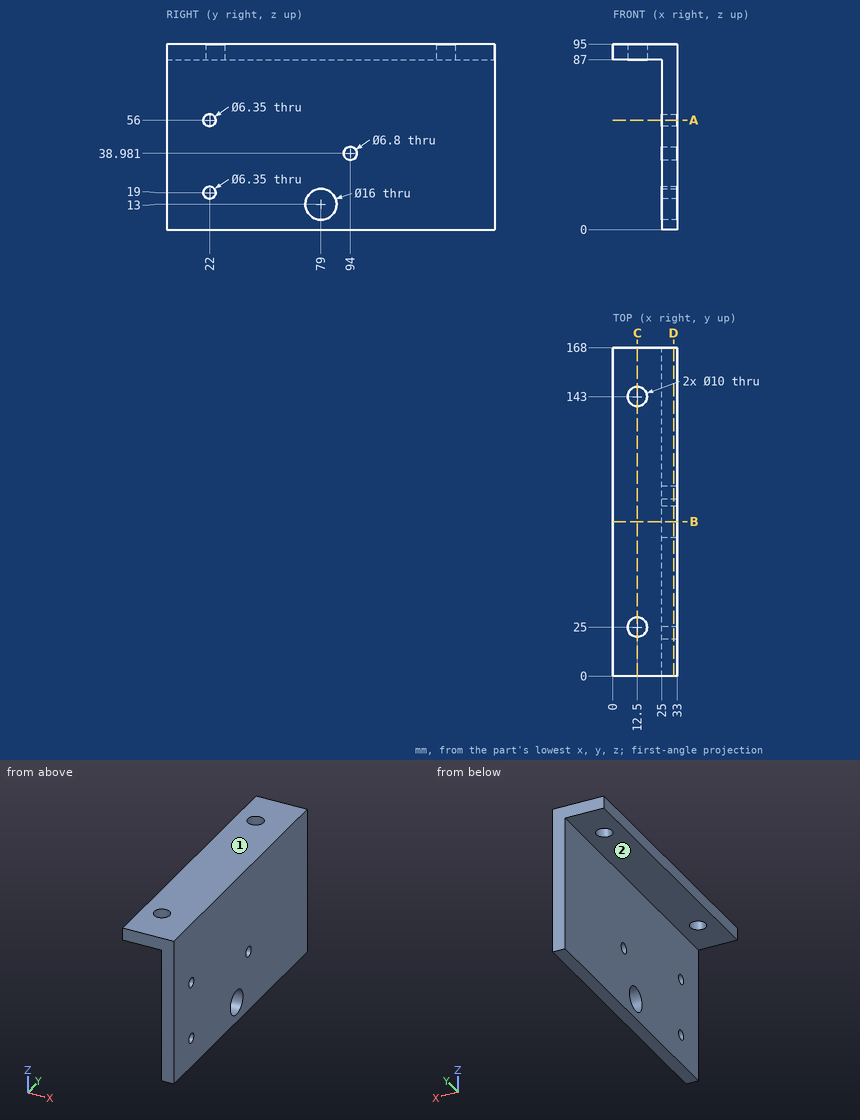
Job drawing, mm, ordinate dimensions from the low corner. One solid piece. A direction names the side the tool comes from. Give positions to 0.01 mm unless a question says otherwise; leave off trailing zeros. Order: outer loops, then holes, each group sorted by start corner. A loop starts at its lowest first (then second) coordinate and runs counter-clockwise, first axis right, second up. Notation, with made-up numbers: (55.5, 15.25) -> (91.5, 15.25) arc R27 cw to (91.5, 39.25) -> close; hole circle Ø8 at (75.25, -11). An arc over 180 degrees is marked (long way). Return JSON: item names as keys, results as strings.
Q1. Saw through at B-B (y = 79). Write the cut outline in (x, z), then the cut area to 3 significant figures.
Working result:
{"outline": "(0, 87) -> (25, 87) -> (25, 21) -> (33, 21) -> (33, 95) -> (0, 95) -> close; (25, 0) -> (33, 0) -> (33, 5) -> (25, 5) -> close", "area": "832 mm²"}
Q2. Drill centre lines: line 1 (Z direction, x = 27.5, y = 22) (3 decimals); line 2 (Y direction, x = 12.5, z = 89.25); line 3 (Y direction, x = 28.25, z = 13). Where is each one in solid material? Low to high.
Working result:
{"line 1": "0 to 15.825, 22.175 to 52.825, 59.175 to 95", "line 2": "0 to 20, 30 to 138, 148 to 168", "line 3": "0 to 71, 87 to 168"}
Q3. Flat gauge pins, fed straight in: pin 1 (21 mm diameter, centred on y = 79, z = 13, fed in from -X); pin 2 (1 mm diameter, centred on x = 18, y = 51, fed in from -Z); pin 3 (6 mm diameter, centred on x = 12.5, y = 25, fed in from -Z). Where does each tip first touch, or does it go through?
Working result:
{"pin 1": "x = 25", "pin 2": "z = 87", "pin 3": "through"}
Q4. Saw through at A-A (z = 56). Write the cut outline in (x, y) (3 decimals).
Working result:
{"outline": "(25, 0) -> (33, 0) -> (33, 18.825) -> (25, 18.825) -> close; (25, 25.175) -> (33, 25.175) -> (33, 168) -> (25, 168) -> close"}
Q5. Saw through at C-C (x = 12.5). Write the cut outline in (y, z).
Working result:
{"outline": "(0, 87) -> (20, 87) -> (20, 95) -> (0, 95) -> close; (30, 87) -> (138, 87) -> (138, 95) -> (30, 95) -> close; (148, 87) -> (168, 87) -> (168, 95) -> (148, 95) -> close"}
Q6. Which spindle directions (+Z, -Z, +X, -X, +Y, -Y) get a long thin tool onto all of the face, cutting with end or side? Do the marked faces 1 and 2. Say none if no direction does.
Working result:
{"face 1": "+Z, +X, -X, +Y, -Y", "face 2": "-Z, -X, +Y, -Y"}
Q7. Saw through at D-D (x = 31). Count the separate pieces of the cut face and the enclosed holes in it, then the cut area to 3 significant figures.
Working result:
{"separate pieces": "1", "enclosed holes": "4", "area": "15,700 mm²"}
